CAD build for the part. Positions are in the model's coordinates, mm. A direction names the side the tool comes from. Round coordinates to 2 decimals unless told otherwise and drop trailing zeros. Write each loop counter-clockwise with the first axis right and the second up, starting at its lowest first coordinate (ties: lowest second). Pieces come first, ordered by that corner, then holes. Notation, with made-up numbers: (30.25, -30.5) - (35.25, -30.5) arc R25 cw to (35.25, 2.5) - close; hole circle Ø7 at (32, 10). An arc over 180 degrees is marked (long way). Put each result on its own line as item: value. Start each with the question number.
Item 1: Cut at A-A (y = 3.5). Give the cut face in (x, z).
Item 2: Pin check, flat tips, straight feed: pin 1 Ø10 at (x, z) = (-35.25, 0) entering from +Y; pin 2 Ø5 at (x, y) = (-24, 17) entering from -Z; pin 3 Ø4 at (x, z) = (-17.5, -24.5) entering from -Y; pin 4 Ø1.5 at (y, z) = (34.5, -34) entering from +X. Stop position of each tip, or through.
Item 3: Drill centre lines: line 1 (Z direction, x = 0, y = 15); line 2 (X direction, y = 47, z = 0); line 3 (Z direction, x = -1, y = 20). Where is each one in solid material? Low to high. Write a range as from..to.
Item 4: 3-axis set-ups, long thin cutter, end or side, ignore diameter. For faces 1 (the flat face through (-23, 50, 22)), 2 (the cylindrical face through (-3.746, 47.535, 35.085)), 3 (the flat face through (32, 5, 32)): which of +Z, -Z, +X, -X, +Y, -Y reach the whole face in a straight line?
Item 5: Cut at B-B (z = -13). Give the cut face in (x, y).
Item 6: Cut at D-D (x = 19.5). Give the cut face in (y, z).
Item 7: Cut at C-C (y = 24.5). Give the cut face in (x, z).
```python
from build123d import *

# Parameters (mm, degrees)
CROQUIS1_R              = 50
CROQUIS1_R_2            = 31.25
SALIENTE_EXTRUIR1_DEPTH = 50
CROQUIS2_R              = 40
CORTAR_EXTRUIR1_DEPTH   = 35
CROQUIS3_R              = 1.5
CORTAR_EXTRUIR2_DEPTH   = 35
CROQUIS3_3_R            = 2
CORTAR_EXTRUIR3_DEPTH   = 51
CROQUIS4_R              = 3.75
CORTAR_EXTRUIR4_DEPTH   = 5
CORTAR_EXTRUIR5_DEPTH   = 5


with BuildPart() as part:
    # Croquis1 → Saliente-Extruir1 (new body)
    with BuildSketch(Plane(origin=(0, 0, 0), x_dir=(1, 0, 0), z_dir=(0, 1, 0))):
        Circle(CROQUIS1_R)
        Circle(CROQUIS1_R_2, mode=Mode.SUBTRACT)
    extrude(amount=SALIENTE_EXTRUIR1_DEPTH)

    # Croquis2 → Cortar-Extruir1 (cut)
    with BuildSketch(Plane.XZ):
        Circle(CROQUIS2_R)
    extrude(amount=-CORTAR_EXTRUIR1_DEPTH, mode=Mode.SUBTRACT)

    # Croquis3 → Cortar-Extruir2 (cut)
    with BuildSketch(Plane.XZ):
        with Locations((0, 45)):
            Circle(CROQUIS3_R)
        with Locations((45, 0)):
            Circle(CROQUIS3_R)
        with Locations((0, -45)):
            Circle(CROQUIS3_R)
        with Locations((-45, 0)):
            Circle(CROQUIS3_R)
    extrude(amount=-CORTAR_EXTRUIR2_DEPTH, mode=Mode.SUBTRACT)

    # Croquis3_3 → Cortar-Extruir3 (cut, through all)
    with BuildSketch(Plane.XZ):
        with Locations((0, 35.25)):
            Circle(CROQUIS3_3_R)
        with Locations((35.25, 0)):
            Circle(CROQUIS3_3_R)
        with Locations((0, -35.25)):
            Circle(CROQUIS3_3_R)
        with Locations((-35.25, 0)):
            Circle(CROQUIS3_3_R)
    extrude(amount=-CORTAR_EXTRUIR3_DEPTH, mode=Mode.SUBTRACT)

    # Croquis4 → Cortar-Extruir4 (cut)
    with BuildSketch(Plane(origin=(0, 50, 0), x_dir=(1, 0, 0), z_dir=(0, 1, 0))):
        with Locations((0, 35.25)):
            Circle(CROQUIS4_R)
        with Locations((35.25, 0)):
            Circle(CROQUIS4_R)
        with Locations((0, -35.25)):
            Circle(CROQUIS4_R)
        with Locations((-35.25, 0)):
            Circle(CROQUIS4_R)
    extrude(amount=-CORTAR_EXTRUIR4_DEPTH, mode=Mode.SUBTRACT)

    # Croquis8 → Cortar-Extruir5 (cut)
    with BuildSketch(Plane.XZ):
        with BuildLine():
            Line((28.284271247, 28.284271247), (35.355339059, 35.355339059))
            ThreePointArc((35.355339059, 35.355339059), (33.541019662, 37.080992435), (31.642584293, 38.713652105))
            Line((31.642584293, 38.713652105), (24.526896495, 31.597964307))
            ThreePointArc((24.526896495, 31.597964307), (26.457513111, 30), (28.284271247, 28.284271247))
        make_face()
        with BuildLine():
            ThreePointArc((38.713652105, 31.642584293), (37.080992435, 33.541019662), (35.355339059, 35.355339059))
            Line((35.355339059, 35.355339059), (28.284271247, 28.284271247))
            ThreePointArc((28.284271247, 28.284271247), (30, 26.457513111), (31.597964307, 24.526896495))
            Line((31.597964307, 24.526896495), (38.713652105, 31.642584293))
        make_face()
    extrude(amount=-CORTAR_EXTRUIR5_DEPTH, mode=Mode.SUBTRACT)


solid = part.part
```
Output values:
1. outline: (24.53, 31.6) - (31.64, 38.71) arc R50 ccw (long way) to (38.71, 31.64) - (31.6, 24.53) arc R40 cw (long way) to start; hole circle Ø3 at (-45, 0); hole circle Ø3 at (0, -45); hole circle Ø3 at (0, 45); hole circle Ø3 at (45, 0)
2. pin 1: y = 50
2. pin 2: z = -45.14
2. pin 3: y = 35
2. pin 4: x = 37.34
3. line 1: -50..-46.5, -43.5..-40, 40..43.5, 46.5..50
3. line 2: -50..-39, -31.5..-31.25, 31.25..31.5, 39..50
3. line 3: -49.99..-46.12, -43.88..-39.99, 39.99..43.88, 46.12..49.99
4. face 1: +Z, -Z, +X, -X, +Y
4. face 2: +Y
4. face 3: -Y
5. outline: (-48.28, 0) - (-37.83, 0) - (-37.83, 35) - (-28.42, 35) - (-28.42, 50) - (-48.28, 50) - close; (28.42, 35) - (37.83, 35) - (37.83, 0) - (48.28, 0) - (48.28, 50) - (28.42, 50) - close
6. outline: (0, -46.04) - (50, -46.04) - (50, -24.42) - (35, -24.42) - (35, -34.92) - (0, -34.92) - close; (0, 34.92) - (35, 34.92) - (35, 24.42) - (50, 24.42) - (50, 46.04) - (0, 46.04) - close
7. outline: circle Ø100 at (0, 0); hole circle Ø3 at (-45, 0); hole circle Ø80 at (0, 0); hole circle Ø3 at (0, -45); hole circle Ø3 at (0, 45); hole circle Ø3 at (45, 0)
